Design review of the part built by this model. Coordinates are the model's own, in mm. A direction names the side the tool comes from. Coordinates: 2 decimals unless noted, no trailing zeros. Write each loop counter-clockwise with the first axis right and the second up, starting at its lowest first coordinate (ties: lowest second). Pieces come first, ordered by that corner, then holes.
Q1. Machinability: for faces 1 (the cylindrical face through (-23.315, 39.805, 3.028)), 2 (the flat face through (-28, -7, -1)), 3 (the flat face through (28, -1, -1)), which of the approach directions +Z, -Z, +X, -X, +Y, -Y give a long, thin tool a straight path to every point of the face, cutting with its end or side? Answer none if there is none.
Q2. Take a section at A-A (x = 21.7). Give the boundary of the cut face in (y, z).
Q3. Insertion check: pin 1 (1 mm diameter, centred on y = 1, z = -1, fed in from +X); pin 2 (4.5 mm diameter, centred on x = 21.7, y = 36.7, fed in from +Z); pin 3 (2 mm diameter, centred on x = 13.5, z = -1.5, fed in from -Y). Each pin has a flat end and moves straight along its axis. Give the tip position at first contact, or say it passes through.
Q4. Take a section at D-D (y = -9). Give the boundary of the cut face in (x, z), and give its area (3 significant figures).
Q5. Take a section at B-B (z = 2.5). Give the boundary of the cut face in (x, y).
Q6. Mouldability with a two-part tool opening along Y and no side actions: class faces 4 (the flat face through (-30, -8, 2)), 5 (the cylindrical face through (-25.49, 40.72, 2.54)), 6 (the flat face through (0, -43, -1)), 7 (the cylindrical face through (-22.775, 35.014, -0.479)) as pulls with the +Y half, pulls with the -Y half, needs draft (parallel to the pull), parting line crosses it, or undercut.
Q7. For probe 1 along Y at (x, z) = (21.7, -1.35); probe 2 along X at (y, z) = (39.5, 4.25); probe 3 along Y at (x, z) = (-21.7, -1.2), list the stretches that pass through material, from the lowest coordinate up.
Q8. Take a section at C-C (y = -36.7). Give the boundary of the cut face in (x, z), and give its area (3 significant figures).
Autodesk Inventor part; units mm, degrees
ref_plane "YZ Plane" through (0, 0, 0) normal (1, 0, 0) x (0, 1, 0)
ref_plane "XZ Plane" through (0, 0, 0) normal (0, 1, 0) x (-1, 0, 0)
ref_plane "XY Plane" through (0, 0, 0) normal (0, 0, 1) x (1, 0, 0)
sketch "Skizze16" plane through (0, 0, 0) normal (0, 0, 1) x (1, 0, 0)
  line L0 (-30, 45) -> (30, 45)
  line L1 (30, 45) -> (30, -45)
  line L2 (30, -45) -> (-30, -45)
  line L3 (-30, -45) -> (-30, 45)
  line L4 (-30, 45) -> (30, -45) construction
  line L5 (30, 45) -> (-30, -45) construction
  point P0 (0, 0)
  dimension "d50" = 60
  dimension "d51" = 90
extrude "Extrusion13" add sketch "Skizze16" along normal blind 5
fillet "Rundung1" radius 15 1 edges at (-30, 45, 2.5)
sketch "Skizze22" plane through (0, 0, 0) normal (0, 0, -1) x (-1, 0, 0)
  line L0 (30, -45) -> (-30, -45)
  line L1 (30, -45) -> (28, -45)
  line L2 (28, -45) -> (28, 30)
  line L3 (28, 30) -> (30, 30)
  line L4 (30, 30) -> (30, -45)
  line L5 (-30, -45) -> (28, -45)
  line L6 (28, -45) -> (28, -43)
  line L7 (28, -43) -> (-30, -43)
  line L8 (-30, -43) -> (-30, -45)
  line L9 (-30, 45) -> (15, 45)
  line L10 (-30, -43) -> (-28, -43)
  line L11 (-28, -43) -> (-28, 45)
  line L12 (-28, 45) -> (-30, 45)
  line L13 (-30, 45) -> (-30, -43)
  line L14 (-28, 45) -> (15, 45)
  line L15 (15, 45) -> (15, 43)
  line L16 (15, 43) -> (-28, 43)
  line L17 (-28, 43) -> (-28, 45)
  arc A0 (30, 30) -> (15, 45) centre (15, 30) ccw
  arc A1 (28, 30) -> (15, 43) centre (15, 30) ccw
  point P0 (0, 0)
  dimension "d92" = 2
  dimension "d93" = 75
  dimension "d94" = 2
  dimension "d95" = 2
  dimension "d96" = 2
extrude "Extrusion17" add sketch "Skizze22" along normal blind 2 contours L7 L11 L16 A1 L2
sketch "Skizze23" plane through (0, 0, 5) normal (0, 0, 1) x (1, 0, 0)
  circle A0 centre (21.7, -36.7) radius 2
  line L0 (30, -45) -> (30, 45)
  line L1 (-30, -45) -> (30, -45)
  point P0 (0, 0)
  dimension "d99" = 4
  dimension "d100" = 8.3
  dimension "d101" = 8.3
extrude "Extrusion18" cut sketch "Skizze23" against normal through all
sketch "Skizze24" plane through (0, 0, 5) normal (0, 0, 1) x (1, 0, 0)
  circle A0 centre (21.7, -36.7) radius 2
  circle A1 centre (21.7, -36.7) radius 3.5
  point P0 (0, 0)
  dimension "d104" = 7
extrude "Extrusion19" cut sketch "Skizze24" against normal blind 4
mirror "Spiegeln5" about plane through (0, 0, 0) normal (0, 1, 0) of "Extrusion19", "Extrusion18"
mirror "Spiegeln6" about plane through (0, 0, 0) normal (1, 0, 0) of "Extrusion19", "Extrusion18", "Spiegeln5"
properties part number "Deckel_Gehäuse"
Response:
1. face 1: +Z
1. face 2: -Z, -X, +Y, -Y
1. face 3: -Z, +X, +Y, -Y
2. outline: (-45, 0) - (-43, 0) - (-43, -2) - (-38.7, -2) - (-38.7, 1) - (-40.2, 1) - (-40.2, 5) - (-45, 5) - close; (-34.7, -2) - (34.7, -2) - (34.7, 1) - (33.2, 1) - (33.2, 5) - (-33.2, 5) - (-33.2, 1) - (-34.7, 1) - close; (38.7, -2) - (43, -2) - (43, 0) - (45, 0) - (45, 5) - (40.2, 5) - (40.2, 1) - (38.7, 1) - close
3. pin 1: stops at x = 28
3. pin 2: stops at z = 1
3. pin 3: stops at y = -43
4. outline: (-30, 0) - (-28, 0) - (-28, -2) - (28, -2) - (28, 0) - (30, 0) - (30, 5) - (-30, 5) - close
4. area: 412 mm2
5. outline: (-30, -45) - (30, -45) - (30, 45) - (-15, 45) arc R15 ccw to (-30, 30) - close; hole circle Ø7 at (-21.7, -36.7); hole circle Ø7 at (-21.7, 36.7); hole circle Ø7 at (21.7, -36.7); hole circle Ø7 at (21.7, 36.7)
6. face 4: needs draft
6. face 5: pulls with the +Y half
6. face 6: pulls with the -Y half
6. face 7: undercut
7. probe 1: y = -43 to -38.7, -34.7 to 34.7, 38.7 to 43
7. probe 2: x = -26.61 to -23.8, -19.6 to 19.6, 23.8 to 30
7. probe 3: y = -43 to -38.7, -34.7 to 34.7, 38.7 to 41.14
8. outline: (-30, 0) - (-28, 0) - (-28, -2) - (-23.7, -2) - (-23.7, 1) - (-25.2, 1) - (-25.2, 5) - (-30, 5) - close; (-19.7, -2) - (19.7, -2) - (19.7, 1) - (18.2, 1) - (18.2, 5) - (-18.2, 5) - (-18.2, 1) - (-19.7, 1) - close; (23.7, -2) - (28, -2) - (28, 0) - (30, 0) - (30, 5) - (25.2, 5) - (25.2, 1) - (23.7, 1) - close
8. area: 332 mm2
